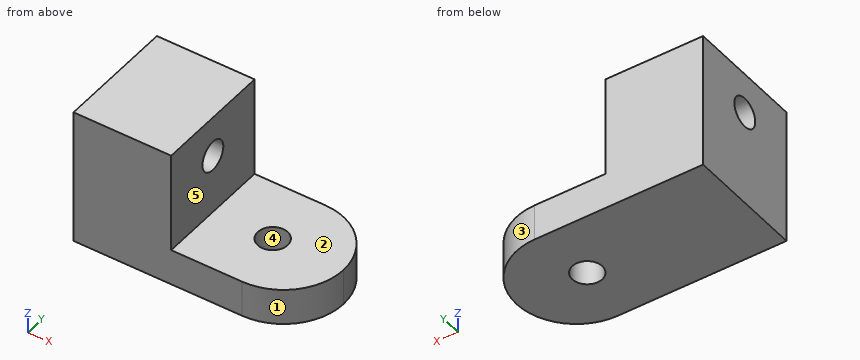
from build123d import *

# Parameters (mm, degrees)
F1_DEPTH = 12.7
F2_R     = 12.69999
F4_D     = 6.35
F6_D     = 6.35


# Not quite as in the source:
# - a fillet or chamfer is up to 0.001 mm smaller than in the source, because OpenCascade refuses the exact size


with BuildPart() as f1:
    # F0 (on Front) → F1 (new body, symmetric)
    with BuildSketch(Plane.XZ):
        Polygon((27.7143083513, 0), (0, 0), (0, 21.3540010154), (-20.7254812121, 21.3540010154), (-20.7254812121, -7.7118072659), (27.7143083513, -7.7118072659), align=None)
    extrude(amount=F1_DEPTH, both=True)

    # F2 (radius 12.7 in the source; OpenCascade refuses exactly that, so slightly less here)
    f2_edges = [f1.edges().sort_by_distance(p)[0] for p in [
        (27.714308, -12.7, -3.855904),
        (27.714308, 12.7, -3.855904),
    ]]
    fillet(f2_edges, radius=F2_R)

    # F4 (through all)
    with Locations(Plane.XY):
        with Locations((12.7, 0)):
            Hole(F4_D / 2)

    # F6 (through all)
    with Locations(Plane.YZ):
        with Locations((0, 12.7)):
            Hole(F6_D / 2)


solid = f1.part
Here's how the part is built. I have some questions about the finished solid (model axes, mm). Face numbers are marked on the shaded views. A direction names the side the tool comes from. Give positions to 0.01 mm unless a question says otherwise; leave off trailing zeros. Loops run counter-clockwise (first coordinate to the right, second up) from the corner with the lowest first, then second, coordinate; pieces in that order, holes last. Notation, with made-up numbers: (70, -21) -> (81, -21) arc R11 ccw to (81, -1) -> close; hole circle Ø5 at (88.25, 0). An arc over 180 degrees is marked (long way). Answer as a JSON object with one key per item and string values. Group by question number.
Item 1: On a 3-axis mill with a long thin cutter (end or side, diameter ignored), from which of +Z, -Z, +X, -X, +Y, -Y can I reach the whole of each face in a straight line? I mean the marked faces 1 and 2. Say none if no direction works.
Item 2: I need wall thicknesses on L1, parallel to Z at x = -9.25, y = 0 (3 decimals); L2, parallel to Y at x = 12.7, z = -4.25 (3 decimals); L3, parallel to Z at x = 5, y = 7.75. Which ranges of each line are inside material? Lowest first, please.
Item 3: Imagine slicing it at C-C on y = -1.25. Write out the boundary of the cut face in (x, z), then the cut area to 3 significant figures.
Item 4: Imagine slicing it at A-A on z = 12.7. Write out the boundary of the cut face in (x, y) (3 decimals).
Item 5: Will these pins go through, and if not, where does the flat tip stop? pin 1 (8 mm diameter, centred on x = 21, z = 3, fed in from +Y); pin 2 (10 mm diameter, centred on x = 12.7, y = 0, fed in from +Z); pin 3 (1 mm diameter, centred on y = -6.5, z = 4, fed in from +X).
Item 6: Imagine slicing it at B-B on x = 12.7. Write out the boundary of the cut face in (y, z) (3 decimals), then the cut area to 3 significant figures.
Item 7: Thinking about a two-plate mould opening in Y: for the marked faces 3, 4 and 5, which applies, pulls with the +Y half, pulls with the -Y half, needs draft (parallel to the pull), parting line crosses it, or undercut?
Answer list:
{
 "1": {"face 1": "+Z, -Z, +X, -Y", "face 2": "+Z, +X, +Y, -Y"},
 "2": {"L1": "z = -7.712 to 9.525, 15.875 to 21.354", "L2": "y = -12.7 to -3.175, 3.175 to 12.7", "L3": "z = -7.71 to 0"},
 "3": {"outline": "(-20.73, -7.71) -> (9.78, -7.71) -> (9.78, 0) -> (0, 0) -> (0, 9.78) -> (-20.73, 9.78) -> close; (-20.73, 15.62) -> (0, 15.62) -> (0, 21.35) -> (-20.73, 21.35) -> close; (15.62, -7.71) -> (27.65, -7.71) -> (27.65, 0) -> (15.62, 0) -> close", "area": "650 mm2"},
 "4": {"outline": "(-20.725, -12.7) -> (0, -12.7) -> (0, -3.175) -> (-20.725, -3.175) -> close; (-20.725, 3.175) -> (0, 3.175) -> (0, 12.7) -> (-20.725, 12.7) -> close"},
 "5": {"pin 1": "stops at y = 12.25", "pin 2": "stops at z = 0", "pin 3": "stops at x = 0"},
 "6": {"outline": "(-12.7, -7.712) -> (-3.175, -7.712) -> (-3.175, 0) -> (-12.7, 0) -> close; (3.175, -7.712) -> (12.7, -7.712) -> (12.7, 0) -> (3.175, 0) -> close", "area": "147 mm2"},
 "7": {"face 3": "pulls with the +Y half", "face 4": "undercut", "face 5": "needs draft"}
}
